Could you check a few things on this model? Use its own coordinates, in mm. Face numbers are marked on the shaded views. A direction names the side the tool comes from. Coordinates: 2 decimals unless noted, no trailing zeros. Write each loop counter-clockwise with the first axis right and the second up, starting at its lowest first coordinate (ties: lowest second). Pieces come first, ordered by that corner, then holes.
```python
from build123d import *

# Parameters (mm, degrees)
BOSS_EXTRUDE1_DEPTH         = 5
FILLET1_R                   = 5
CUT_EXTRUDE1_DEPTH          = 10
F_3_0MM_DOWEL_HOLE3_D       = 3
CUT_EXTRUDE2_DEPTH          = 5
F_3_0MM_PRESS_DOWEL_HOLE1_D = 3
F_5_0MM_PRESS_DOWEL_HOLE1_D = 5


with BuildPart() as part:
    # Sketch1 → Boss-Extrude1 (new, symmetric)
    with BuildSketch(Plane(origin=(0, 0, 0), x_dir=(1, 0, 0), z_dir=(0, 1, 0))):
        with BuildLine():
            Line((-107.462553071, 24.023952891), (-41.71930009, -41.71930009))
            ThreePointArc((-41.71930009, -41.71930009), (3.806502253, -58.877079926), (46.74398357, -36))
            Line((46.74398357, -36), (84.4, -36))
            Line((84.4, -36), (84.4, 36))
            Line((84.4, 36), (46.74398357, 36))
            ThreePointArc((46.74398357, 36), (26.048032555, 52.93864373), (0, 59))
            Line((0, 59), (-110.83863918, 62.740943777))
            Line((-110.83863918, 62.740943777), (-128.004005064, 44.565404884))
            Line((-128.004005064, 44.565404884), (-107.462553071, 24.023952891))
        make_face()
        with BuildLine():
            Line((49, 14.576290822), (46.781745862, 14.576290822))
            ThreePointArc((46.781745862, 14.576290822), (-49, 0), (46.781745862, -14.576290822))
            Line((46.781745862, -14.576290822), (49, -14.576290822))
            Line((49, -14.576290822), (49, 14.576290822))
        make_face(mode=Mode.SUBTRACT)
        with BuildLine():
            Line((-93.296148974, 23.999684418), (-57.886132355, -11.410332201))
            ThreePointArc((-57.886132355, -11.410332201), (-57.048958802, 15.047135926), (-44.728269399, 38.475731527))
            Line((-44.728269399, 38.475731527), (-78.820101865, 38.475731527))
            Line((-78.820101865, 38.475731527), (-93.296148974, 23.999684418))
        make_face(mode=Mode.SUBTRACT)
    extrude(amount=BOSS_EXTRUDE1_DEPTH, both=True)

    # Fillet1
    # the kernel refuses this fillet: 5 mm, written as the material it adds along each edge
    with BuildSketch(Plane(origin=(46.74398357, -5, 36), x_dir=(1, 0, 0), z_dir=(0, 1, 0))) as fillet1_piece_1:
        with BuildLine():
            CenterArc((2.398665931, -5), FILLET1_R, 90, 50.161560023)
            ThreePointArc((-1.440603561, -1.796875), (-0.711533327, -0.905467408), (0, 0))
            Line((0, 0), (2.398665931, 0))
        make_face()
    extrude(amount=10)
    with BuildSketch(Plane(origin=(46.74398357, -5, -36), x_dir=(-0.6255163967442842, 0, -0.7802110210731757), z_dir=(0, 1, 0))) as fillet1_piece_2:
        with BuildLine():
            CenterArc((2.400650235, -4.999047579), FILLET1_R, 91.118340331, 50.161560023)
            Line((-1.50040487, -1.871465595), (0, 0))
            ThreePointArc((0, 0), (1.151531414, -0.011238567), (2.303062827, 0))
        make_face()
    extrude(amount=10)
    with BuildSketch(Plane(origin=(-93.296148974, -5, -23.999684418), x_dir=(0.7071067811865481, 0, -0.7071067811865468), z_dir=(0, 1, 0))) as fillet1_piece_3:
        with BuildLine():
            CenterArc((FILLET1_R, -FILLET1_R), FILLET1_R, 90, 90)
            Line((0, -FILLET1_R), (0, 0))
            Line((0, 0), (FILLET1_R, 0))
        make_face()
    extrude(amount=10)
    with BuildSketch(Plane(origin=(-78.820101865, -5, -38.475731527), x_dir=(1, 0, 0), z_dir=(0, 1, 0))) as fillet1_piece_4:
        with BuildLine():
            CenterArc((FILLET1_R * 0.414213562373, -FILLET1_R), FILLET1_R, 90, 45)
            Line((-FILLET1_R * 0.292893218813, -FILLET1_R * 0.292893218813), (0, 0))
            Line((0, 0), (FILLET1_R * 0.414213562373, 0))
        make_face()
    extrude(amount=10)
    with BuildSketch(Plane(origin=(-57.886132355, 5, 11.410332201), x_dir=(-0.08353472888006676, 0, -0.9965048665565731), z_dir=(0, -1, 0))) as fillet1_piece_5:
        with BuildLine():
            CenterArc((13.623707644, -4.969234882), FILLET1_R, 96.359234778, 133.432536558)
            Line((10.395870767, -8.787751491), (0, 0))
            ThreePointArc((0, 0), (6.534949195, -0.363028395), (13.06989839, 0))
        make_face()
    extrude(amount=10)
    with BuildSketch(Plane(origin=(-44.728269399, -5, -38.475731527), x_dir=(-0.5894789818981541, 0, 0.807783714802617), z_dir=(0, 1, 0))) as fillet1_piece_6:
        with BuildLine():
            CenterArc((9.826854917, -4.984017175), FILLET1_R, 94.582422839, 121.53762105)
            Line((5.787936343, -7.931412084), (0, 0))
            ThreePointArc((0, 0), (4.713694635, -0.18859734), (9.42738927, 0))
        make_face()
    extrude(amount=10)
    # the kernel refuses this fillet: 5 mm, written as the material it takes off along each edge
    with BuildSketch(Plane(origin=(46.781745862, 12.95259813, 14.576290822), x_dir=(-0.32830869078175484, 0, 0.9445704862831413), z_dir=(0, -1, 0)), Plane(origin=(46.781745862, -12.95259813, -14.576290822), x_dir=(-0.32830869078175745, 0, -0.9445704862831404), z_dir=(0, 1, 0))) as fillet1_2_piece_1:
        with BuildLine():
            CenterArc((3.343337173, -4.997365244), FILLET1_R, 91.860123923, 52.660239811)
            Line((-0.728272112, -2.09529739), (0, 0))
            ThreePointArc((0, 0), (1.590519626, -0.025820606), (3.181039252, 0))
        make_face()
    extrude(amount=25.90519626, mode=Mode.SUBTRACT)
    with BuildSketch(Plane(origin=(-110.83863918, 10.640073082, -62.740943777), x_dir=(-0.6866146353868613, 0, 0.7270215557138366), z_dir=(0, -1, 0))) as fillet1_2_piece_2:
        with BuildLine():
            CenterArc((FILLET1_R * 0.451205846565, -FILLET1_R), FILLET1_R, 90, 48.570349235)
            Line((-FILLET1_R * 0.298562891452, -FILLET1_R * 0.338300038165), (0, 0))
            Line((0, 0), (FILLET1_R * 0.451205846565, 0))
        make_face()
    extrude(amount=21.280146164, mode=Mode.SUBTRACT)

    # Sketch11 → Cut-Extrude1 (cut)
    with BuildSketch(Plane(origin=(-41.71930009, 0, 41.71930009), x_dir=(0.7071067811865458, 0, 0.7071067811865492), z_dir=(-0.7071067811865492, 0, 0.7071067811865458))):
        Polygon((-116.963470882, 5), (-116.963470882, 2.5), (-119.963470882, 2.5), (-119.963470882, -2.5), (-84.963470882, -2.5), (-84.963470882, 2.5), (-87.963470882, 2.5), (-87.963470882, 5), align=None)
    extrude(amount=-CUT_EXTRUDE1_DEPTH, mode=Mode.SUBTRACT)

    # Ø3.0mm Dowel Hole3 (through all)
    with Locations(Plane(origin=(-113.995138479, -2.5, -37.627606111), x_dir=(0, 0, 1), z_dir=(0, 1, 0))):
        with Locations((0, 0), (6.717514421, 6.717514421)):
            Hole(F_3_0MM_DOWEL_HOLE3_D / 2)

    # Sketch33 → Cut-Extrude2 (cut)
    with BuildSketch(Plane(origin=(0, 5, 0), x_dir=(1, 0, 0), z_dir=(0, 1, 0))):
        Polygon((59, 19.5), (59, -19.5), (54, -19.5), (54, -14.576290822), (49, -14.576290822), (49, 14.576290822), (54, 14.576290822), (54, 19.5), align=None)
    extrude(amount=-CUT_EXTRUDE2_DEPTH, mode=Mode.SUBTRACT)

    # Ø3.0mm Press Dowel Hole1 (through all)
    with Locations(Plane(origin=(53.32762779, -5, -4.850211912), x_dir=(0, 0, -1), z_dir=(0, -1, 0))):
        with Locations((0, 0), (-9.700423824, 0)):
            Hole(F_3_0MM_PRESS_DOWEL_HOLE1_D / 2)

    # Ø5.0mm Press Dowel Hole1 (through all)
    with Locations(Plane(origin=(71.7, 5, 24.5), x_dir=(0, 0, 1), z_dir=(0, 1, 0))):
        with Locations((0, 0), (-49, 0)):
            Hole(F_5_0MM_PRESS_DOWEL_HOLE1_D / 2)


solid = part.part
```
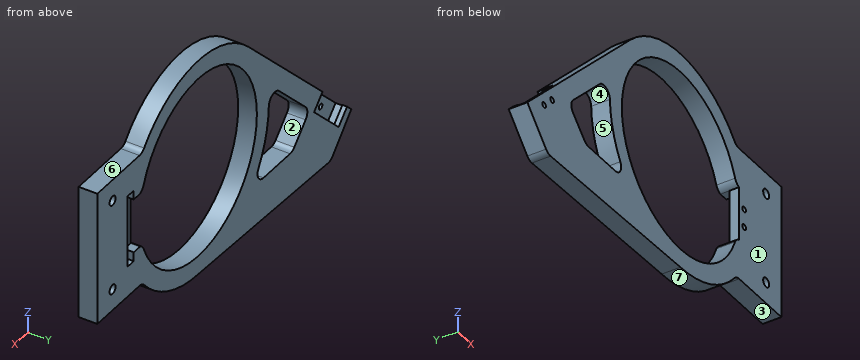
1. I want a section at A-A on x = 31. Please give me the cut outline in (y, z), plus the area to 3 significant figures.
Verdict:
outline: (-5, -50.2) - (5, -50.2) - (5, -37.95) - (-5, -37.95) - close; (-5, 37.95) - (5, 37.95) - (5, 50.2) - (-5, 50.2) - close
area: 245 mm2
2. On a 3-axis mill with a long thin cutter (end or side, diameter ignored), from which of +Z, -Z, +X, -X, +Y, -Y can I reach the whole of each face in a straight line? I mean the marked faces 1, 2 and 3. Say none if no direction works.
Verdict:
face 1: +Z, -Z, +X, -X, -Y
face 2: +Y, -Y
face 3: -Z, +X, +Y, -Y
3. I want a section at C-C on z = 24.5. Please give me the cut outline in (x, y).
Verdict:
outline: (-58.94, -5) - (-42.44, -5) - (-42.44, 5) - (-58.94, 5) - close; (42.44, -5) - (69.2, -5) - (69.2, 5) - (42.44, 5) - close; (74.2, -5) - (84.4, -5) - (84.4, 5) - (74.2, 5) - close
4. If we mould it in two halves opening along X, with no side actions, what happens to the marked faces 4, 5, 6 and 7? For each: pulls with the +X half, pulls with the -X half, needs draft (parallel to the pull), parting line crosses it, or undercut.
Verdict:
face 4: undercut
face 5: undercut
face 6: needs draft
face 7: pulls with the +X half
5. I want a section at D-D on x = -64. Please give me the cut outline in (y, z).
Verdict:
outline: (-5, -61.16) - (5, -61.16) - (5, -38.48) - (-5, -38.48) - close; (-5, 3.25) - (5, 3.25) - (5, 19.44) - (-5, 19.44) - close
6. Please list where these lines run through material, in increasing order: line 1 along X through (y, z) = (2, -30.5); line 2 along X through (y, z) = (-1, -24.5); line 3 along X through (y, z) = (0, -26).
Verdict:
line 1: x = -99.8 to -86.8, -50.5 to -38.35, 38.35 to 84.4
line 2: x = -95.66 to -91.2, -53.67 to -42.44, 42.44 to 69.2, 74.2 to 84.4
line 3: x = -95.3 to -90.81, -52.96 to -41.53, 41.53 to 69.7, 73.7 to 84.4
7. For pin 1 (3.5 mm diameter, centred on x = -107.28, z = -30.91, fed in from +Y); pin 2 (1 mm diameter, centred on y = 3, z = 37, fed in from -X); pin 3 (4 mm diameter, centred on x = 57.5, y = 3, fed in from +Z); pin 4 (1.8 mm diameter, centred on x = 53.33, z = -4.85, fed in from +Y), each with a flat end and sliding along its axis, tell me the tip position at first contact or that it passes through.
Verdict:
pin 1: stops at y = -2.5
pin 2: stops at x = -46.94
pin 3: stops at z = 36
pin 4: passes through
8. I want a section at B-B on x = 71.7. Please give me the cut outline in (y, z), plus the area to 3 significant figures.
Verdict:
outline: (-5, -36) - (5, -36) - (5, -27) - (-5, -27) - close; (-5, -22) - (5, -22) - (5, 22) - (-5, 22) - close; (-5, 27) - (5, 27) - (5, 36) - (-5, 36) - close
area: 620 mm2
